```python
from build123d import *

# Parameters (mm, degrees)
F0_W      = 63.5
F0_H      = 38.1
F0_R      = 3.96875
F1_DEPTH  = 15.24
F3_DEPTH  = 7.62
F4_R      = 5.08
F5_DEPTH  = 3.81
F7_DEPTH  = 25.4
F8_R      = 6.35
F8_R_2    = 3.81
F9_DEPTH  = 7.62
F11_D     = 6.7564
F11_DEPTH = 16.51
F11_TIP   = 2.0298273432
F13_D     = 12.7
F13_DEPTH = 3.81
F13_TIP   = 3.8154649308
F14_R     = 2.54


with BuildPart() as f1:
    # F0 (on Front) → F1 (new body)
    with BuildSketch(Plane.XZ):
        Rectangle(F0_W, F0_H)
        with Locations((-23.8125, -11.1252)):
            Circle(F0_R, mode=Mode.SUBTRACT)
        with Locations((23.8125, -11.1125)):
            Circle(F0_R, mode=Mode.SUBTRACT)
        with Locations((-23.8125, 11.1125)):
            Circle(F0_R, mode=Mode.SUBTRACT)
        with Locations((23.8125, 11.1125)):
            Circle(F0_R, mode=Mode.SUBTRACT)
    extrude(amount=F1_DEPTH)

    # F2 (on face) → F3 (cut)
    with BuildSketch(Plane.XZ.offset(15.24)):
        with BuildLine():
            ThreePointArc((10.16, -10.16), (17.3442048969, -7.1842048969), (20.32, 0))
            ThreePointArc((20.32, 0), (17.3442048969, 7.1842048969), (10.16, 10.16))
            ThreePointArc((10.16, 10.16), (2.9757951031, 7.1842048969), (0, 0))
            ThreePointArc((0, 0), (2.9757951031, -7.1842048969), (10.16, -10.16))
        make_face()
        with BuildLine():
            ThreePointArc((0, 0), (2.9757951031, 7.1842048969), (10.16, 10.16))
            Line((10.16, 10.16), (-10.16, 10.16))
            ThreePointArc((-10.16, 10.16), (-2.9757951031, 7.1842048969), (0, 0))
        make_face()
        with BuildLine():
            Line((-10.16, -10.16), (10.16, -10.16))
            ThreePointArc((10.16, -10.16), (2.9757951031, -7.1842048969), (0, 0))
            ThreePointArc((0, 0), (-2.9757951031, -7.1842048969), (-10.16, -10.16))
        make_face()
        with BuildLine():
            ThreePointArc((-10.16, -10.16), (-2.9757951031, -7.1842048969), (0, 0))
            ThreePointArc((0, 0), (-2.9757951031, 7.1842048969), (-10.16, 10.16))
            ThreePointArc((-10.16, 10.16), (-20.32, 0), (-10.16, -10.16))
        make_face()
    extrude(amount=-F3_DEPTH, mode=Mode.SUBTRACT)

    # F4 (on face) → F5 (cut)
    with BuildSketch(Plane.XZ.offset(7.62)):
        with Locations((10.16, 0)):
            Circle(F4_R)
    extrude(amount=-F5_DEPTH, mode=Mode.SUBTRACT)

    # F6 (on face) → F7 (cut)
    with BuildSketch(Plane.XZ.offset(15.24)):
        with BuildLine():
            ThreePointArc((-3.81, 10.16), (0, 6.35), (3.81, 10.16))
            Line((3.81, 10.16), (-3.81, 10.16))
        make_face()
        with BuildLine():
            Line((-3.81, 10.16), (3.81, 10.16))
            ThreePointArc((3.81, 10.16), (0, 13.97), (-3.81, 10.16))
        make_face()
    extrude(amount=-F7_DEPTH, mode=Mode.SUBTRACT)

    # F8 (on face) → F9 (cut)
    with BuildSketch(Plane(origin=(0, 0, 0), x_dir=(-1, 0, 0), z_dir=(0, 1, 0))):
        with Locations((0, 10.16)):
            Circle(F8_R)
        with Locations((0, 10.16)):
            Circle(F8_R_2, mode=Mode.SUBTRACT)
    extrude(amount=-F9_DEPTH, mode=Mode.SUBTRACT)

    # F11
    with Locations(Plane(origin=(0, 0, -19.05), x_dir=(1, 0, 0), z_dir=(0, 0, -1))):
        with Locations((0, 7.62)):
            Hole(F11_D / 2, depth=F11_DEPTH)
            with Locations((0, 0, -(F11_DEPTH + F11_TIP / 2))):  # 118° drill point
                Cone(0, F11_D / 2, F11_TIP, mode=Mode.SUBTRACT)

    # F13
    with Locations(Plane(origin=(0, 0, -19.05), x_dir=(1, 0, 0), z_dir=(0, 0, -1))):
        with Locations((0, 7.62)):
            Hole(F13_D / 2, depth=F13_DEPTH)
            with Locations((0, 0, -(F13_DEPTH + F13_TIP / 2))):  # 118° drill point
                Cone(0, F13_D / 2, F13_TIP, mode=Mode.SUBTRACT)

    # F14
    f14_edges = [f1.edges().sort_by_distance(p)[0] for p in [
        (31.75, -7.62, -19.05),
        (-31.75, -7.62, -19.05),
        (31.75, -7.62, 19.05),
        (-31.75, -7.62, 19.05),
    ]]
    fillet(f14_edges, radius=F14_R)


solid = f1.part
```
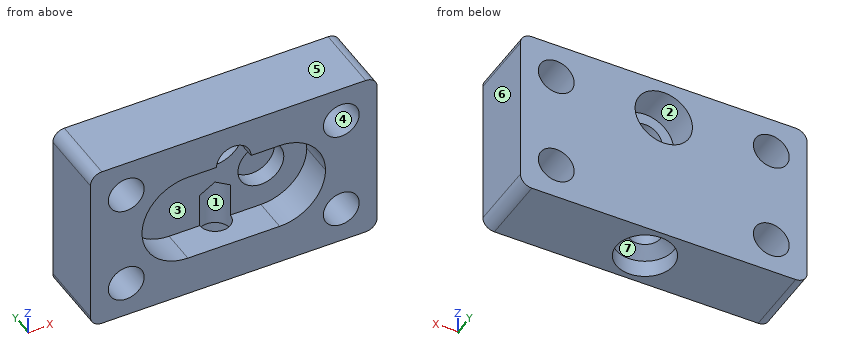
The model under review builds one solid part; all positions refer to its coordinate system, in mm. Face numbers are marked on the shaded views. A direction names the side the tool comes from. Coordinates: 2 decimals unless noted, no trailing zeros. Write each loop counter-clockwise with the first axis right and the second up, starting at its lowest first coordinate (ties: lowest second). Pieces come first, ordered by that corner, then holes. Notation, with made-up numbers: (53.5, -29) - (60.5, -29) arc R29 cw to (60.5, 10) - close; hole circle Ø4 at (62.25, 57.25). An arc over 180 degrees is marked (long way). Answer in a Markdown table with one row per item. Add a question column.
Q1. Consider section B-B on z = 9. Give the boundary of the cut face in (x, y), then the cut area to 3 significant figures.
Q2. Consider section A-A on x = 0. Give the boundary of the cut face in (y, z).
Q3. For the marked faces 1, 2 and 3, list the 3-axis set-ups (+Z, -Z, +X, -X, +Y, -Y) from which the entire face can be reached by the end or side of a thin tool; tool diameter is ignored.
Q4. To check wall thickness, follow line 1 along Z through (x, y) = (-23.5, -4.75); line 2 along X through (y, z) = (-1, 11); line 3 along Z through (x, y) = (-24.5, -9.25). State the ranges of each line that lie inside material, in increasing order. Write a range as from..to.
Q5. Consider section C-C on z = -8.5. Give the boundary of the cut face in (x, y), then the cut area to 3 significant figures.
Q6. Consider section D-D on y = -11.75. Give the number of separate pieces and of enclosed holes in the cut face, then the cut area to 3 significant figures.
Q7. Clearance check with flat-ended pins moving along their axes: pin 1 (5 mm diameter, centred on x = 9, z = 1.5, fed in from -Y); pin 2 (4 mm diameter, centred on x = -2, z = 5.5, fed in from -Y); pin 3 (3 mm diameter, centred on x = 1.5, z = 13.5, fed in from +Y). State where each tip first meets the part, or that it passes through.
Q8. Draft analysis for pull direction Z (two halves, no side actions). For the marked faces 4, 5, 6 and 7, state which applies: +Z half, -Z half, draft (parallel to the pull), parting line (faces both ways), or undercut.
Answers below:
| question | item | result |
|---|---|---|
| 1 | outline | (-31.75, -15.24) - (-27.17, -15.24) - (-27.17, 0) - (-31.75, 0) - close; (-20.45, -15.24) - (-14.87, -15.24) - (-14.87, -7.62) - (-6.24, -7.62) - (-6.24, 0) - (-20.45, 0) - close; (6.24, -7.62) - (14.87, -7.62) - (14.87, -15.24) - (20.45, -15.24) - (20.45, 0) - (6.24, 0) - close; (27.17, -15.24) - (31.75, -15.24) - (31.75, 0) - (27.17, 0) - close |
| 1 | area | 441 mm² |
| 2 | outline | (-15.24, -19.05) - (-13.97, -19.05) - (-13.97, -15.24) - (-11, -13.45) - (-11, -10.16) - (-15.24, -10.16) - close; (-15.24, 13.97) - (-7.62, 13.97) - (-7.62, 16.51) - (0, 16.51) - (0, 19.05) - (-15.24, 19.05) - close; (-7.62, -0.51) - (-4.24, -2.54) - (-4.24, -13.45) - (-1.27, -15.24) - (-1.27, -19.05) - (0, -19.05) - (0, 3.81) - (-7.62, 3.81) - close |
| 3 | face 1 | -Z |
| 3 | face 2 | +Y |
| 3 | face 3 | -Y |
| 4 | line 1 | -19.05..-15.08, -7.17..7.16, 15.07..19.05 |
| 4 | line 2 | -31.75..-27.78, -19.85..-6.29, 6.29..19.85, 27.78..31.75 |
| 4 | line 3 | -19.05..-15.03, -7.22..7.2, 15.02..19.05 |
| 5 | outline | (-31.75, -15.24) - (-26.79, -15.24) - (-26.79, 0) - (-31.75, 0) - close; (-20.84, -15.24) - (-15.73, -15.24) - (-15.73, -7.62) - (-3.38, -7.62) arc R3.38 cw to (3.38, -7.62) - (15.73, -7.62) - (15.73, -15.24) - (20.82, -15.24) - (20.82, 0) - (-20.84, 0) - close; (26.8, -15.24) - (31.75, -15.24) - (31.75, 0) - (26.8, 0) - close |
| 5 | area | 528 mm² |
| 6 | separate pieces | 1 |
| 6 | enclosed holes | 5 |
| 6 | area | 1,410 mm² |
| 7 | pin 1 | y = -3.81 |
| 7 | pin 2 | y = -7.62 |
| 7 | pin 3 | y = -7.62 |
| 8 | face 4 | undercut |
| 8 | face 5 | +Z half |
| 8 | face 6 | draft |
| 8 | face 7 | -Z half |
